```python
from build123d import *

# Parameters (mm, degrees)
ESBO_O9_R                         = 1.250000058
ESBO_O9_R_2                       = 1.250559391
RESSALTO_EXTRUS_O2_DEPTH          = 24
CORTE_EXTRUS_O5_DEPTH             = 28.088973642
CORTE_EXTRUS_O5_DEPTH_BACK        = 28.088973642
ESBO_O12_OUTSIDE_W                = 60.428
ESBO_O12_OUTSIDE_H                = 20.928
CORTE_EXTRUS_O6_REACH             = 29.089
ESBO_O13_W                        = 3.805227374
ESBO_O13_H                        = 1.999999904
ESBO_O13_W_2                      = 36.154186404
ESBO_O13_H_2                      = 31.243547385
ESBO_O13_H_3                      = 1.961388226
CORTE_EXTRUS_O6_DIRECTION_2_DEPTH = 5000


with BuildPart() as part:
    # Esboço9 → Ressalto-extrusão2 (new, symmetric)
    with BuildSketch(Plane(origin=(0, 0, 0), x_dir=(0, 0, -1), z_dir=(1, 0, 0))):
        with BuildLine():
            Line((0, -5.999999999), (0, 5.999999999))
            Line((0, 5.999999999), (-1.714464294, 6.00000012))
            Line((-1.714464294, 6.00000012), (-4.232231545, 8.517767251))
            ThreePointArc((-4.232231545, 8.517767251), (-6.956707169, 9.059699215), (-8.499999099, 6.7500006))
            Line((-8.499999099, 6.7500006), (-8.499999099, -6.749999877))
            ThreePointArc((-8.499999099, -6.749999877), (-7.153358538, -8.968070124), (-4.564293582, -8.794809974))
            Line((-4.564293582, -8.794809974), (-1.714465141, -5.999999999))
            Line((-1.714465141, -5.999999999), (0, -5.999999999))
        make_face()
        with Locations((-5.999998683, 6.749999894)):
            Circle(ESBO_O9_R, mode=Mode.SUBTRACT)
        with Locations((-6.001403792, -6.750869293)):
            Circle(ESBO_O9_R_2, mode=Mode.SUBTRACT)
    extrude(amount=RESSALTO_EXTRUS_O2_DEPTH, both=True)

    # Esboço12 outside → Corte-extrusão5 (cut, two sides: drawn at the far end of the back side and taken through both)
    with BuildSketch(Plane(origin=(0, 0, 0), x_dir=(1, 0, 0), z_dir=(0, 1, 0)).offset(-CORTE_EXTRUS_O5_DEPTH_BACK)):
        with Locations((0, -4.25)):
            Rectangle(ESBO_O12_OUTSIDE_W, ESBO_O12_OUTSIDE_H)
        Polygon((-24, -4), (-24, 0), (24, 0), (24, -4), (20.194772626, -4), (20.194772626, -2), (14, -2), (14, -9.171977472), (6, -9.171977472), (6, -2), (-6, -2), (-6, -9.171977472), (-14, -9.171977472), (-14, -2), (-20.194772626, -2), (-20.194772626, -4), align=None, mode=Mode.SUBTRACT)
    extrude(amount=CORTE_EXTRUS_O5_DEPTH + CORTE_EXTRUS_O5_DEPTH_BACK, mode=Mode.SUBTRACT)

    # Corte-extrusão6: up to this face of the body (flat: up to its plane)
    corte_extrus_o6_end = Plane(part.part.faces().sort_by_distance((-17.097386313, 0.002756729, 2))[0])
    # Esboço13 → Corte-extrusão6 (cut, up to the picked face)
    with BuildSketch(Plane.XY.offset(8.499999099), mode=Mode.PRIVATE) as corte_extrus_o6_sk1:
        with Locations((-22.097386313, 7.285535765)):
            Rectangle(ESBO_O13_W, ESBO_O13_H)
    corte_extrus_o6_tool1 = split(extrude(corte_extrus_o6_sk1.sketch, amount=-CORTE_EXTRUS_O6_REACH, mode=Mode.PRIVATE), bisect_by=corte_extrus_o6_end, keep=Keep.BOTH, mode=Mode.PRIVATE)
    # Esboço13 → Corte-extrusão6 (cut, up to the picked face)
    with BuildSketch(Plane.XY.offset(8.499999099), mode=Mode.PRIVATE) as corte_extrus_o6_sk2:
        with Locations((-0.25062362, -2.463016757)):
            Rectangle(ESBO_O13_W_2, ESBO_O13_H_2)
        Polygon((-14, 9.25000031), (-14, 2.75000031), (-9.75, -2.749464751), (-9.75, -9.249464751), (-6, -9.249464751), (-6, -2.749464751), (-10.25, 2.75000031), (-10.25, 9.25000031), align=None, mode=Mode.SUBTRACT)
        Polygon((6, -2.749464751), (6, -9.249464751), (9.75, -9.249464751), (9.75, -2.749464751), (14, 2.75000031), (14, 9.25000031), (10.25, 9.25000031), (10.25, 2.75000031), align=None, mode=Mode.SUBTRACT)
    corte_extrus_o6_tool2 = split(extrude(corte_extrus_o6_sk2.sketch, amount=-CORTE_EXTRUS_O6_REACH, mode=Mode.PRIVATE), bisect_by=corte_extrus_o6_end, keep=Keep.BOTH, mode=Mode.PRIVATE)
    # Esboço13 → Corte-extrusão6 (cut, up to the picked face)
    with BuildSketch(Plane.XY.offset(8.499999099), mode=Mode.PRIVATE) as corte_extrus_o6_sk3:
        with Locations((-22.097386313, -7.260716467)):
            Rectangle(ESBO_O13_W, ESBO_O13_H_3)
    corte_extrus_o6_tool3 = split(extrude(corte_extrus_o6_sk3.sketch, amount=-CORTE_EXTRUS_O6_REACH, mode=Mode.PRIVATE), bisect_by=corte_extrus_o6_end, keep=Keep.BOTH, mode=Mode.PRIVATE)
    # Esboço13 → Corte-extrusão6 (cut, up to the picked face)
    with BuildSketch(Plane.XY.offset(8.499999099), mode=Mode.PRIVATE) as corte_extrus_o6_sk4:
        with Locations((22.097386313, 7.285535765)):
            Rectangle(ESBO_O13_W, ESBO_O13_H)
    corte_extrus_o6_tool4 = split(extrude(corte_extrus_o6_sk4.sketch, amount=-CORTE_EXTRUS_O6_REACH, mode=Mode.PRIVATE), bisect_by=corte_extrus_o6_end, keep=Keep.BOTH, mode=Mode.PRIVATE)
    # Esboço13 → Corte-extrusão6 (cut, up to the picked face)
    with BuildSketch(Plane.XY.offset(8.499999099), mode=Mode.PRIVATE) as corte_extrus_o6_sk5:
        with Locations((22.097386313, -7.260716467)):
            Rectangle(ESBO_O13_W, ESBO_O13_H_3)
    corte_extrus_o6_tool5 = split(extrude(corte_extrus_o6_sk5.sketch, amount=-CORTE_EXTRUS_O6_REACH, mode=Mode.PRIVATE), bisect_by=corte_extrus_o6_end, keep=Keep.BOTH, mode=Mode.PRIVATE)
    add(corte_extrus_o6_tool1.solids().sort_by(Axis((-22.097386, 7.285536, 8.499999), (0, 0, -1)))[0], mode=Mode.SUBTRACT)
    add(corte_extrus_o6_tool2.solids().sort_by(Axis((-0.285718, -2.807947, 8.499999), (0, 0, -1)))[0], mode=Mode.SUBTRACT)
    add(corte_extrus_o6_tool3.solids().sort_by(Axis((-22.097386, -7.260716, 8.499999), (0, 0, -1)))[0], mode=Mode.SUBTRACT)
    add(corte_extrus_o6_tool4.solids().sort_by(Axis((22.097386, 7.285536, 8.499999), (0, 0, -1)))[0], mode=Mode.SUBTRACT)
    add(corte_extrus_o6_tool5.solids().sort_by(Axis((22.097386, -7.260716, 8.499999), (0, 0, -1)))[0], mode=Mode.SUBTRACT)

    # Esboço13 → Corte-extrusão6 direction 2 (cut)
    # profile 1 of 5: a face of its own
    with BuildSketch(Plane.XY.offset(8.499999099)):
        with Locations((-22.097386313, 7.285535765)):
            Rectangle(ESBO_O13_W, ESBO_O13_H)
    # profile 2 of 5: a face of its own
    with BuildSketch(Plane.XY.offset(8.499999099)):
        with Locations((-0.25062362, -2.463016757)):
            Rectangle(ESBO_O13_W_2, ESBO_O13_H_2)
        Polygon((-14, 9.25000031), (-14, 2.75000031), (-9.75, -2.749464751), (-9.75, -9.249464751), (-6, -9.249464751), (-6, -2.749464751), (-10.25, 2.75000031), (-10.25, 9.25000031), align=None, mode=Mode.SUBTRACT)
        Polygon((6, -2.749464751), (6, -9.249464751), (9.75, -9.249464751), (9.75, -2.749464751), (14, 2.75000031), (14, 9.25000031), (10.25, 9.25000031), (10.25, 2.75000031), align=None, mode=Mode.SUBTRACT)
    # profile 3 of 5: a face of its own
    with BuildSketch(Plane.XY.offset(8.499999099)):
        with Locations((-22.097386313, -7.260716467)):
            Rectangle(ESBO_O13_W, ESBO_O13_H_3)
    # profile 4 of 5: a face of its own
    with BuildSketch(Plane.XY.offset(8.499999099)):
        with Locations((22.097386313, 7.285535765)):
            Rectangle(ESBO_O13_W, ESBO_O13_H)
    # profile 5 of 5: a face of its own
    with BuildSketch(Plane.XY.offset(8.499999099)):
        with Locations((22.097386313, -7.260716467)):
            Rectangle(ESBO_O13_W, ESBO_O13_H_3)
    extrude(amount=CORTE_EXTRUS_O6_DIRECTION_2_DEPTH, mode=Mode.SUBTRACT)


solid = part.part
```
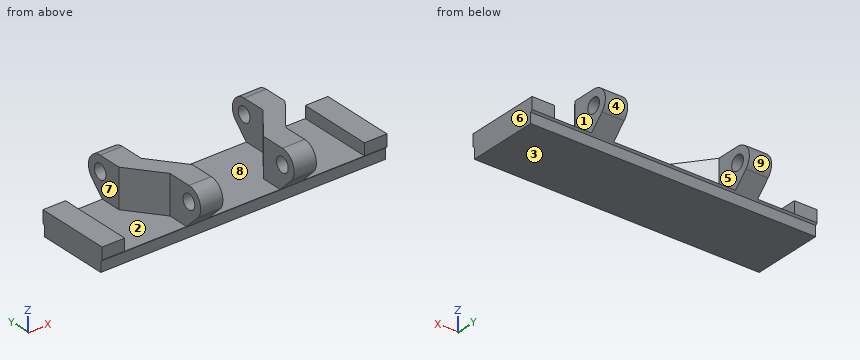
Model file for the job. Use its own axes, mm. Face numbers are marked on the shaded views. A direction names the side the tool comes from. Coordinates: 2 decimals unless noted, no trailing zeros. Write each loop counter-clockwise with the first axis right and the second up, starting at its lowest first coordinate (ties: lowest second). Pieces come first, ordered by that corner, then holes. Notation, with made-up numbers: (16.5, -17.75) - (36.5, -17.75) arc R18 ccw to (36.5, 12.25) - close; hole circle Ø9 at (-32, 50.25). An arc over 180 degrees is marked (long way). Use a Markdown table: item, result. Add a question column.
Item 1: Two-plate mould, pull along X, no slides. Class the marked faces 6, 7, 8 and 9: pulls with the +X half, pulls with the -X half, needs draft (parallel to the pull), parting line crosses it, or undercut.
Item 2: Band-saw the part on D-D, the plane z = 6.5. Give the number of separate pieces and of enclosed holes in the cut face, and give its area (3 significant figures).
Item 3: Drill centre lines: line 1 along X through (y, z) = (-3.75, 2.75); line 2 along X through (y, z) = (3, 3.25); line 3 along X through (y, z) = (4.75, 8.25). Where is each one in solid material? Low to high.
Item 4: 3-axis set-ups, long thin cutter, end or side, ignore diameter. For the marked faces 1, 2, 3, 4 and 5: which of +Z, -Z, +X, -X, +Y, -Y reach the whole face in a straight line?
Item 5: Band-saw the part on B-B, the plane x = 18. Write the cut outline in (y, z).
Item 6: Band-saw the part on C-C, the plane y = 4. Write the cut outline in (x, z).
Item 7: Drop flat-ended pins along their axis: pin 1 (1.9 mm diameter, centred on x = 23, y = -0.5, fed in from +Z); pin 2 (6 mm diameter, centred on x = 1.5, y = -2, fed in from +Z); pin 3 (1.5 mm diameter, centred on y = -3, z = 7.5, fed in from +X); pin 4 (5 mm diameter, centred on x = 13, y = -0.5, fed in from +Z). Give the stop position or say it passes through.
Item 8: Band-saw the part on A-A, the plane z = 3.5. Write the cut outline in (x, y).
A:
| question | item | result |
|---|---|---|
| 1 | face 6 | pulls with the +X half |
| 1 | face 7 | undercut |
| 1 | face 8 | undercut |
| 1 | face 9 | needs draft |
| 2 | separate pieces | 6 |
| 2 | enclosed holes | 0 |
| 2 | area | 104 mm² |
| 3 | line 1 | x = -24 to -20.19, -9.75 to -6, 6 to 9.75, 20.19 to 24 |
| 3 | line 2 | x = -24 to -20.19, -14 to -10.25, 10.25 to 14, 20.19 to 24 |
| 3 | line 3 | x = -14 to -10.25, 10.25 to 14 |
| 4 | face 1 | +Z, +Y, -Y |
| 4 | face 2 | +Z, -Y |
| 4 | face 3 | -Z, +X, -X, +Y, -Y |
| 4 | face 4 | +X, -X, +Y |
| 4 | face 5 | +Z, +Y |
| 5 | outline | (-6.28, 2) - (-6, 1.71) - (-6, 0) - (6, 0) - (6, 1.71) - (6.29, 2) - close |
| 6 | outline | (-24, 0) - (24, 0) - (24, 4) - (20.19, 4) - (20.19, 2) - (14, 2) - (14, 8.5) - (10.25, 8.5) - (10.25, 2) - (-10.25, 2) - (-10.25, 8.5) - (-14, 8.5) - (-14, 2) - (-20.19, 2) - (-20.19, 4) - (-24, 4) - close |
| 7 | pin 1 | stops at z = 4 |
| 7 | pin 2 | stops at z = 2 |
| 7 | pin 3 | stops at x = 10.14 |
| 7 | pin 4 | stops at z = 8.5 |
| 8 | outline | (-24, -6.28) - (-20.19, -6.28) - (-20.19, 6.29) - (-24, 6.29) - close; (-14, 2.75) - (-9.75, -2.75) - (-9.75, -7.75) - (-6, -7.75) - (-6, -2.75) - (-10.25, 2.75) - (-10.25, 7.79) - (-14, 7.79) - close; (6, -7.75) - (9.75, -7.75) - (9.75, -2.75) - (14, 2.75) - (14, 7.79) - (10.25, 7.79) - (10.25, 2.75) - (6, -2.75) - close; (20.19, -6.28) - (24, -6.28) - (24, 6.29) - (20.19, 6.29) - close |
